The listing builds one solid part. Answer for the finished solid, in the listing's coordinates (mm). Face numbers are marked on the shaded views. A direction names the side the tool comes from. Coordinates: 2 decimals unless noted, no trailing zeros. Loops run counter-clockwise (first coordinate to the right, second up) from the corner with the lowest first, then second, coordinate; pieces in that order, holes last. Notation, with made-up numbers: (-28.5, 26.5) - (-21.5, 26.5) arc R30 ccw to (-21.5, 64.5) - close; hole circle Ø6 at (88, 45). An arc over 180 degrees is marked (long way). Return JSON: item names as keys, results as strings. Group by question number.
1. The mould has two halves that part along Z. Classify the marked faces 3, 4 and 5: pulls with the +Z half, pulls with the -Z half, needs draft (parallel to the pull), parting line crosses it, or undercut.
2. Section B-B (x = 1) is taken. Write down the section's boundary in (y, z) (3 decimals).
3. Section A-A (y = -7.62) is taken. Write down the section's boundary in (x, z) (3 decimals).
4. Each of these flat-tipped pins is pushed along its axis until it touches: P1, Ø3, axis at y = 5, z = -3, coming from the +X side; P2, Ø2.5, axis at x = 5, y = -4, coming from the -Z side; P3, Ø2, axis at y = -1, z = -1.5, coming from the -X side (3 decimals). Where does it stop, or does it pass through?
5. Find the intervals of material crossed by line 1 along Y through (x, z) = (0, -2.75); line 2 along Y through (x, z) = (0.75, -3); line 3 along X through (y, z) = (7.5, 1.25), in increasing order.
6. Which of the six approach directions +Z, -Z, +X, -X, +Y, -Y give full straight-line access (tool end or side, diameter ignored) to the marked faces 1 and 2?
7. Section C-C (y = -4.5) is taken. Write down the section's boundary in (x, z) (3 decimals), and give its area (3 significant figures).
8. Section D-D (z = 1.25) is taken. Write down the section's boundary in (x, y).
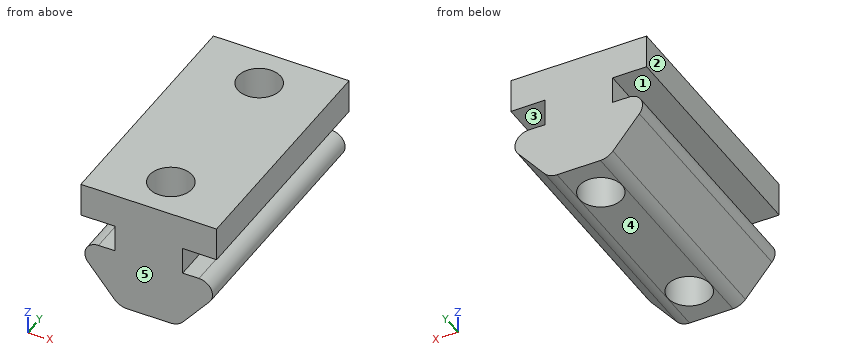
```python
from build123d import *

# Parameters (mm, degrees)
SKETCH1_W           = 12.7
SKETCH1_H           = 22.86
BOSS_EXTRUDE1_DEPTH = 3.175
BOSS_EXTRUDE2_DEPTH = 22.86
SKETCH4_R           = 2
CUT_EXTRUDE1_DEPTH  = 18.283668852


with BuildPart() as part:
    # Sketch1 → Boss-Extrude1 (new body)
    with BuildSketch(Plane.XY):
        Rectangle(SKETCH1_W, SKETCH1_H)
    extrude(amount=BOSS_EXTRUDE1_DEPTH)

    # Sketch2 → Boss-Extrude2 (add)
    with BuildSketch(Plane(origin=(0, 11.43, 0), x_dir=(1, 0, 0), z_dir=(0, 1, 0))):
        with BuildLine():
            Line((3.175, 0), (3.175, 2.54))
            Line((3.175, 2.54), (4.699372999, 2.54))
            ThreePointArc((4.699372999, 2.54), (5.849922417, 3.272286288), (5.673650477, 4.624667659))
            Line((5.673650477, 4.624667659), (3.201132974, 7.581601191))
            ThreePointArc((3.201132974, 7.581601191), (2.677256455, 7.984659302), (2.032, 8.128))
            Line((2.032, 8.128), (-2.032, 8.128))
            ThreePointArc((-2.032, 8.128), (-2.677256455, 7.984659302), (-3.201132974, 7.581601191))
            Line((-3.201132974, 7.581601191), (-5.673650477, 4.624667659))
            ThreePointArc((-5.673650477, 4.624667659), (-5.849922417, 3.272286288), (-4.699372999, 2.54))
            Line((-4.699372999, 2.54), (-3.175, 2.54))
            Line((-3.175, 2.54), (-3.175, 0))
            Line((-3.175, 0), (3.175, 0))
        make_face()
    extrude(amount=-BOSS_EXTRUDE2_DEPTH)

    # Sketch4 → Cut-Extrude1 (cut, through all)
    with BuildSketch(Plane.XY.offset(3.175)):
        with Locations((0, 7.62)):
            Circle(SKETCH4_R)
        with Locations((0, -7.62)):
            Circle(SKETCH4_R)
    extrude(amount=-CUT_EXTRUDE1_DEPTH, mode=Mode.SUBTRACT)


solid = part.part
```
The answers:
{
 "1": {"face 3": "undercut", "face 4": "pulls with the -Z half", "face 5": "needs draft"},
 "2": {"outline": "(-11.43, -8.128) - (-9.352, -8.128) - (-9.352, 3.175) - (-11.43, 3.175) - close; (-5.888, -8.128) - (5.888, -8.128) - (5.888, 3.175) - (-5.888, 3.175) - close; (9.352, -8.128) - (11.43, -8.128) - (11.43, 3.175) - (9.352, 3.175) - close"},
 "3": {"outline": "(-6.35, 0) - (-3.175, 0) - (-3.175, -2.54) - (-4.699, -2.54) arc R1.27 ccw to (-5.674, -4.625) - (-3.201, -7.582) arc R1.524 ccw to (-2.032, -8.128) - (-2, -8.128) - (-2, 3.175) - (-6.35, 3.175) - close; (2, -8.128) - (2.032, -8.128) arc R1.524 ccw to (3.201, -7.582) - (5.674, -4.625) arc R1.27 ccw to (4.699, -2.54) - (3.175, -2.54) - (3.175, 0) - (6.35, 0) - (6.35, 3.175) - (2, 3.175) - close"},
 "4": {"P1": "stops at x = 5.97", "P2": "stops at z = -6.93", "P3": "stops at x = -3.175"},
 "5": {"line 1": "y = -11.43 to -9.62, -5.62 to 5.62, 9.62 to 11.43", "line 2": "y = -11.43 to -9.47, -5.77 to 5.77, 9.47 to 11.43", "line 3": "x = -6.35 to -2, 2 to 6.35"},
 "6": {"face 1": "-X, +Y, -Y", "face 2": "+Z, -Z, -X, +Y, -Y"},
 "7": {"outline": "(-6.35, 0) - (-3.175, 0) - (-3.175, -2.54) - (-4.699, -2.54) arc R1.27 ccw to (-5.674, -4.625) - (-3.201, -7.582) arc R1.524 ccw to (-2.032, -8.128) - (2.032, -8.128) arc R1.524 ccw to (3.201, -7.582) - (5.674, -4.625) arc R1.27 ccw to (4.699, -2.54) - (3.175, -2.54) - (3.175, 0) - (6.35, 0) - (6.35, 3.175) - (-6.35, 3.175) - close", "area": "110 mm2"},
 "8": {"outline": "(-6.35, -11.43) - (6.35, -11.43) - (6.35, 11.43) - (-6.35, 11.43) - close; hole circle Ø4 at (0, -7.62); hole circle Ø4 at (0, 7.62)"}
}
